Geometry: final body of the model. Coordinates: model frame, mm. A direction names the side the tool comes from. Give positions to 0.01 mm unless a question says otherwise; leave off trailing zeros. Write each loop counter-clockwise with the first axis right and the second up, starting at its lowest first coordinate (ties: lowest second). Pieces come first, ordered by that corner, then holes. Notation, with made-up numbers: M 20.5,80.25 L 64.5,80.25 A24 ccw 64.5,91.25 Z; hole C -21.75,28.5 d10. An arc over 180 degrees is marked long. Answer as a JSON object with one key per item and string values.
from build123d import *

# Parameters (mm, degrees)
SKETCH1_R           = 37.5
BOSS_EXTRUDE1_DEPTH = 10
SKETCH2_R           = 9.59
CUT_EXTRUDE1_DEPTH  = 10


with BuildPart() as part:
    # Sketch1 → Boss-Extrude1 (new body)
    with BuildSketch(Plane(origin=(0, 0, 0), x_dir=(1, 0, 0), z_dir=(0, 1, 0))):
        Circle(SKETCH1_R)
        with BuildLine():
            ThreePointArc((-14.404165277, 34.623258406), (-11.588137289, 35.664619361), (-8.697826179, 36.477360373))
            Line((-8.697826179, 36.477360373), (-11.506647359, 43.503989088))
            Line((-11.506647359, 43.503989088), (-16.26192994, 41.958904116))
            Line((-16.26192994, 41.958904116), (-14.404165277, 34.623258406))
        make_face()
        with BuildLine():
            ThreePointArc((-24.398350496, 28.477543663), (-22.041946961, 30.338137289), (-19.54424853, 32.004255176))
            Line((-19.54424853, 32.004255176), (-24.386943903, 37.819002725))
            Line((-24.386943903, 37.819002725), (-28.432028874, 34.880076463))
            Line((-28.432028874, 34.880076463), (-24.398350496, 28.477543663))
        make_face()
        with BuildLine():
            ThreePointArc((-32.004255176, 19.54424853), (-30.338137289, 22.041946961), (-28.477543663, 24.398350496))
            Line((-28.477543663, 24.398350496), (-34.880076463, 28.432028874))
            Line((-34.880076463, 28.432028874), (-37.819002725, 24.386943903))
            Line((-37.819002725, 24.386943903), (-32.004255176, 19.54424853))
        make_face()
        with BuildLine():
            ThreePointArc((-36.477360373, 8.697826179), (-35.664619361, 11.588137289), (-34.623258406, 14.404165277))
            Line((-34.623258406, 14.404165277), (-41.958904116, 16.26192994))
            Line((-41.958904116, 16.26192994), (-43.503989088, 11.506647359))
            Line((-43.503989088, 11.506647359), (-36.477360373, 8.697826179))
        make_face()
        with BuildLine():
            ThreePointArc((-37.379807383, -3), (-37.5, 0), (-37.379807383, 3))
            Line((-37.379807383, 3), (-44.930501889, 2.5))
            Line((-44.930501889, 2.5), (-44.930501889, -2.5))
            Line((-44.930501889, -2.5), (-37.379807383, -3))
        make_face()
        with BuildLine():
            ThreePointArc((-34.623258406, -14.404165277), (-35.664619361, -11.588137289), (-36.477360373, -8.697826179))
            Line((-36.477360373, -8.697826179), (-43.503989088, -11.506647359))
            Line((-43.503989088, -11.506647359), (-41.958904116, -16.26192994))
            Line((-41.958904116, -16.26192994), (-34.623258406, -14.404165277))
        make_face()
        with BuildLine():
            ThreePointArc((-28.477543663, -24.398350496), (-30.338137289, -22.041946961), (-32.004255176, -19.54424853))
            Line((-32.004255176, -19.54424853), (-37.819002725, -24.386943903))
            Line((-37.819002725, -24.386943903), (-34.880076463, -28.432028874))
            Line((-34.880076463, -28.432028874), (-28.477543663, -24.398350496))
        make_face()
        with BuildLine():
            ThreePointArc((-19.54424853, -32.004255176), (-22.041946961, -30.338137289), (-24.398350496, -28.477543663))
            Line((-24.398350496, -28.477543663), (-28.432028874, -34.880076463))
            Line((-28.432028874, -34.880076463), (-24.386943903, -37.819002725))
            Line((-24.386943903, -37.819002725), (-19.54424853, -32.004255176))
        make_face()
        with BuildLine():
            ThreePointArc((-8.697826179, -36.477360373), (-11.588137289, -35.664619361), (-14.404165277, -34.623258406))
            Line((-14.404165277, -34.623258406), (-16.26192994, -41.958904116))
            Line((-16.26192994, -41.958904116), (-11.506647359, -43.503989088))
            Line((-11.506647359, -43.503989088), (-8.697826179, -36.477360373))
        make_face()
        with BuildLine():
            ThreePointArc((3, -37.379807383), (0, -37.5), (-3, -37.379807383))
            Line((-3, -37.379807383), (-2.5, -44.930501889))
            Line((-2.5, -44.930501889), (2.5, -44.930501889))
            Line((2.5, -44.930501889), (3, -37.379807383))
        make_face()
        with BuildLine():
            Line((11.506647359, -43.503989088), (16.26192994, -41.958904116))
            Line((16.26192994, -41.958904116), (14.404165277, -34.623258406))
            ThreePointArc((14.404165277, -34.623258406), (11.588137289, -35.664619361), (8.697826179, -36.477360373))
            Line((8.697826179, -36.477360373), (11.506647359, -43.503989088))
        make_face()
        with BuildLine():
            Line((24.386943903, -37.819002725), (28.432028874, -34.880076463))
            Line((28.432028874, -34.880076463), (24.398350496, -28.477543663))
            ThreePointArc((24.398350496, -28.477543663), (22.041946961, -30.338137289), (19.54424853, -32.004255176))
            Line((19.54424853, -32.004255176), (24.386943903, -37.819002725))
        make_face()
        with BuildLine():
            Line((34.880076463, -28.432028874), (37.819002725, -24.386943903))
            Line((37.819002725, -24.386943903), (32.004255176, -19.54424853))
            ThreePointArc((32.004255176, -19.54424853), (30.338137289, -22.041946961), (28.477543663, -24.398350496))
            Line((28.477543663, -24.398350496), (34.880076463, -28.432028874))
        make_face()
        with BuildLine():
            Line((41.958904116, -16.26192994), (43.503989088, -11.506647359))
            Line((43.503989088, -11.506647359), (36.477360373, -8.697826179))
            ThreePointArc((36.477360373, -8.697826179), (35.664619361, -11.588137289), (34.623258406, -14.404165277))
            Line((34.623258406, -14.404165277), (41.958904116, -16.26192994))
        make_face()
        with BuildLine():
            Line((44.930501889, 2.5), (37.379807383, 3))
            ThreePointArc((37.379807383, 3), (37.469939798, 1.501203373), (37.5, 0))
            ThreePointArc((37.5, 0), (37.469939798, -1.501203373), (37.379807383, -3))
            Line((37.379807383, -3), (44.930501889, -2.5))
            Line((44.930501889, -2.5), (44.930501889, 2.5))
        make_face()
        with BuildLine():
            Line((41.958904116, 16.26192994), (34.623258406, 14.404165277))
            ThreePointArc((34.623258406, 14.404165277), (35.664619361, 11.588137289), (36.477360373, 8.697826179))
            Line((36.477360373, 8.697826179), (43.503989088, 11.506647359))
            Line((43.503989088, 11.506647359), (41.958904116, 16.26192994))
        make_face()
        with BuildLine():
            Line((34.880076463, 28.432028874), (28.477543663, 24.398350496))
            ThreePointArc((28.477543663, 24.398350496), (30.338137289, 22.041946961), (32.004255176, 19.54424853))
            Line((32.004255176, 19.54424853), (37.819002725, 24.386943903))
            Line((37.819002725, 24.386943903), (34.880076463, 28.432028874))
        make_face()
        with BuildLine():
            Line((24.386943903, 37.819002725), (19.54424853, 32.004255176))
            ThreePointArc((19.54424853, 32.004255176), (22.041946961, 30.338137289), (24.398350496, 28.477543663))
            Line((24.398350496, 28.477543663), (28.432028874, 34.880076463))
            Line((28.432028874, 34.880076463), (24.386943903, 37.819002725))
        make_face()
        with BuildLine():
            Line((11.506647359, 43.503989088), (8.697826179, 36.477360373))
            ThreePointArc((8.697826179, 36.477360373), (11.588137289, 35.664619361), (14.404165277, 34.623258406))
            Line((14.404165277, 34.623258406), (16.26192994, 41.958904116))
            Line((16.26192994, 41.958904116), (11.506647359, 43.503989088))
        make_face()
        with BuildLine():
            Line((-2.5, 44.930501889), (-3, 37.379807383))
            ThreePointArc((-3, 37.379807383), (0, 37.5), (3, 37.379807383))
            Line((3, 37.379807383), (2.5, 44.930501889))
            Line((2.5, 44.930501889), (-2.5, 44.930501889))
        make_face()
    extrude(amount=BOSS_EXTRUDE1_DEPTH)

    # Sketch2 → Cut-Extrude1 (cut)
    with BuildSketch(Plane(origin=(0, 10, 0), x_dir=(1, 0, 0), z_dir=(0, 1, 0))):
        with Locations(Location((0, 0, 0), (0, 0, 270))):
            Circle(SKETCH2_R)
    extrude(amount=-CUT_EXTRUDE1_DEPTH, mode=Mode.SUBTRACT)


solid = part.part
1) Line query: line 1 (X direction, y = 4.5, z = 0); line 2 (X direction, y = 7.5, z = -25); line 3 (X direction, y = 0.75, z = 35.5). Output: solid intervals per line, ascending. Write a range as from..to.
Geometry check:
{"line 1": "x = -44.93..-9.59, 9.59..44.93", "line 2": "x = -37.37..-29.43, -27.95..27.95, 29.43..37.37", "line 3": "x = -27.58..-22.46, -14.63..14.63, 22.46..27.58"}
2) Set-up query: faces 1 (the flat face through (-26.44, 4.93, -31.72)), 2 (the flat face through (-31.634, 4.93, -26.387)), 3 (the cylindrical face through (5.826, 4.93, 37.045)). Return all of +Z, -Z, +X, -X, +Y, -Y with unobstructed straight access to the full face (end or side cutting, diameter ignored); none if empty.
Geometry check:
{"face 1": "-X, +Y, -Y", "face 2": "-Z, +Y, -Y", "face 3": "+Z, +Y, -Y"}
3) Cut plane C-C on z = 39. Return loops of the section in (x, y).
Geometry check:
{"outline": "M -15.51,0 L -9.71,0 L -9.71,10 L -15.51,10 Z; M -2.89,0 L 2.89,0 L 2.89,10 L -2.89,10 Z; M 9.71,0 L 15.51,0 L 15.51,10 L 9.71,10 Z"}
4) Cut plane D-D on z = 13. Return loops of the section in (x, y).
Geometry check:
{"outline": "M -43.02,0 L 43.02,0 L 43.02,10 L -43.02,10 Z"}
5) Cut plane B-B on z = 0. Return loops of the section in (x, y).
Geometry check:
{"outline": "M -44.93,0 L -9.59,0 L -9.59,10 L -44.93,10 Z; M 9.59,0 L 44.93,0 L 44.93,10 L 9.59,10 Z"}
6) Cut plane A-A on x = 0. Return loops of the section in (y, z).
Geometry check:
{"outline": "M 0,-44.93 L 10,-44.93 L 10,-9.59 L 0,-9.59 Z; M 0,9.59 L 10,9.59 L 10,44.93 L 0,44.93 Z"}
7) Contact query for flat-ended pins moving along their axis: P1, Ø1.5, axis at x = 28.5, z = 22, coming from the -Y side; P2, Ø1.5, axis at x = 23.5, y = 1, coming from the +Z side; P3, Ø1.5, axis at x = -12, y = 4.5, coming from the -Z side. Output: stop coordinate, or through.
Geometry check:
{"P1": "stops at y = 0", "P2": "stops at z = 37.65", "P3": "stops at z = -43.5"}
8) Pull-direction query (Z, two-part tool) for faces 4 (the flat face through (-10.08, 4.93, -39.94)), 5 (the flat face through (13.851, 4.93, 42.742)), 6 (the flat face through (41.208, 4.93, -2.746)); classes: pulls with the +Z half, pulls with the -Z half, needs draft (parallel to the pull), parting line crosses it, or undercut.
Geometry check:
{"face 4": "pulls with the -Z half", "face 5": "pulls with the +Z half", "face 6": "undercut"}
